Autodesk Inventor part; units mm, degrees
ref_plane "YZ Plane" through (0, 0, 0) normal (1, 0, 0) x (0, 1, 0)
ref_plane "XZ Plane" through (0, 0, 0) normal (0, 1, 0) x (-1, 0, 0)
ref_plane "XY Plane" through (0, 0, 0) normal (0, 0, 1) x (1, 0, 0)
sketch "Sketch1" plane through (0, 0, 0) normal (0, 0, 1) x (1, 0, 0)
  line L0 (2.8868, 0) -> (1.4434, -2.5)
  line L1 (1.4434, -2.5) -> (-1.4434, -2.5)
  line L2 (-1.4434, -2.5) -> (-2.8868, 0)
  line L3 (-2.8868, 0) -> (-1.4434, 2.5)
  line L4 (-1.4434, 2.5) -> (1.4434, 2.5)
  line L5 (1.4434, 2.5) -> (2.8868, 0)
  point P0 (0, 0)
  point P1 (0, 0)
  dimension "d0" = 5
extrude "Extrusion1" add sketch "Sketch1" along normal blind 20
sketch "Sketch3" plane through (0, 0, 0) normal (0, 0, -1) x (-1, 0, 0)
  circle A0 centre (0, 0) radius 1.25
  dimension "d6" = 2.5
extrude "Extrusion3" cut sketch "Sketch3" against normal through all
properties part number "M2.5x12mm_Standoff_ 971120151"
CAD build for the part. Positions are in the model's coordinates, mm. Round coordinates to 2 decimals unless told otherwise and drop trailing zeros. Write each loop counter-clockwise with the first axis right and the second up, starting at its lowest first coordinate (ties: lowest second). Pieces come first, ordered by that corner, then holes. Notation, with made-up numbers: (-39, -14.5) - (-16, -14.5) arc R17 ccw to (-16, -1.5) - close; hole circle Ø8 at (-14.75, -34). An arc over 180 degrees is marked (long way). Return JSON: item names as keys, results as strings. Group by question number.
Item 1: Band-saw the part on D-D on y = -1.9. List the corners of the cut face in (x, z).
Item 2: Mould opens along X. For faces 1 (the face through (0.27, -1.22, 9.86)), 2 (the face through (0, -2.5, 10)), 3 (the face through (-2.175, 1.233, 9.86)) say: +X half, -X half, draft (parallel to the pull), parting line (faces both ways), or undercut.
Item 3: Flat gauge pins, fed straight in: pin 1 Ø3 at (y, z) = (1, 3) entering from +X; pin 2 Ø1 at (x, z) = (-2, 13) entering from -Y. Where does each tip first touch, or does it go through?
Item 4: Band-saw the part on C-C on y = -0.6. List the corners of the cut face in (x, z), plus the area to 3 significant figures.
Item 5: Band-saw the part on A-A on x = 0. List the corners of the cut face in (y, z).
Item 6: Band-saw the part on B-B on z = 11.25. List the corners of the cut face in (x, y).
Item 7: Probe probe 1 along Y at (x, z) = (-0.1, 8); probe 2 along Y at (x, z) = (-1.1, 10.5); probe 3 along X at (y, z) = (0.75, 5). List the from-to ranges inside material, lowest first.
Resolved:
{
 "1": {"outline": "(-1.79, 0) - (1.79, 0) - (1.79, 20) - (-1.79, 20) - close"},
 "2": {"face 1": "undercut", "face 2": "draft", "face 3": "-X half"},
 "3": {"pin 1": "stops at x = 2.89", "pin 2": "stops at y = -2.4"},
 "4": {"outline": "(-2.54, 0) - (-1.1, 0) - (-1.1, 20) - (-2.54, 20) - close; (1.1, 0) - (2.54, 0) - (2.54, 20) - (1.1, 20) - close", "area": "57.8 mm²"},
 "5": {"outline": "(-2.5, 0) - (-1.25, 0) - (-1.25, 20) - (-2.5, 20) - close; (1.25, 0) - (2.5, 0) - (2.5, 20) - (1.25, 20) - close"},
 "6": {"outline": "(-2.89, 0) - (-1.44, -2.5) - (1.44, -2.5) - (2.89, 0) - (1.44, 2.5) - (-1.44, 2.5) - close; hole circle Ø2.5 at (0, 0)"},
 "7": {"probe 1": "y = -2.5 to -1.25, 1.25 to 2.5", "probe 2": "y = -2.5 to -0.59, 0.59 to 2.5", "probe 3": "x = -2.45 to -1, 1 to 2.45"}
}
